Source: three-view drawing plus pictorial views. Frame: mm from the lowest corner of the part. A direction names the side the tool comes from. Give positions to 0.01 mm unless a question says otherwise; leave off trailing zeros. Write each loop counter-clockwise with the first axis right and the second up, starting at its lowest first coordinate (ties: lowest second). Pieces come first, ordered by that corner, then holes. Notation, with made-up numbers: (65.5, 1.25) -> (108.5, 1.25) arc R25 cw to (108.5, 32.25) -> close; hole circle Ø3 at (85.25, 75). An arc over 180 degrees is marked (long way). Write item = value, one per line.
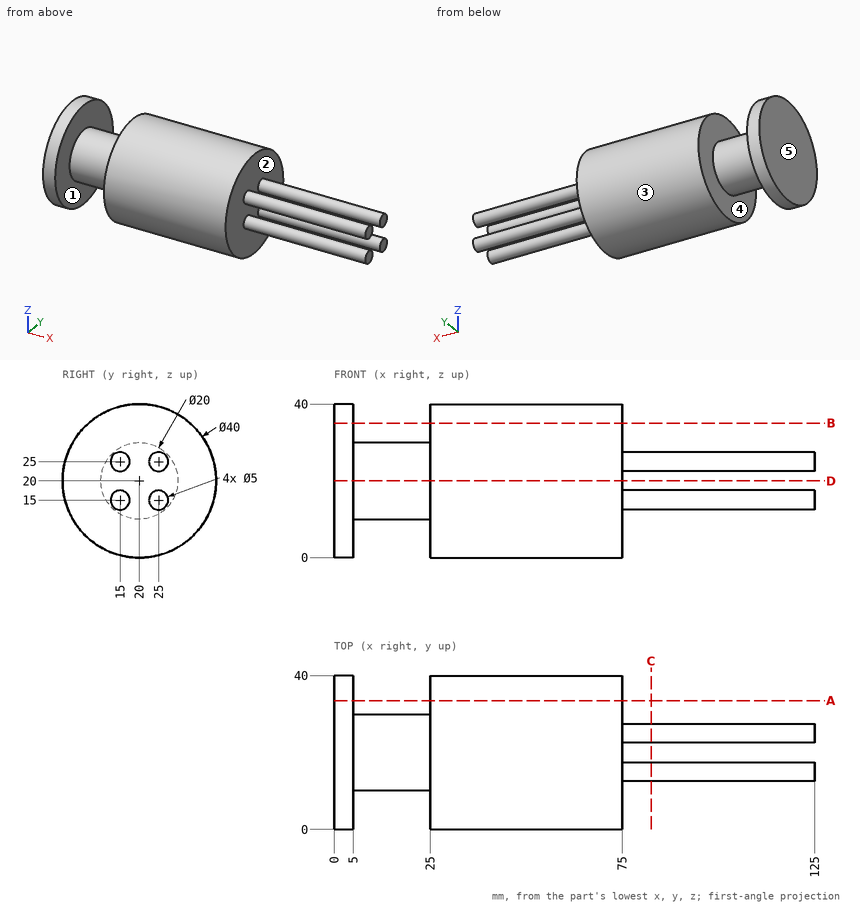
1) Draft query along X for the marked faces 1, 2 and 3. Return one class per face: pulls with the +X half, pulls with the -X half, needs draft (parallel to the pull), parting line crosses it, or undercut.
Computed:
face_1 = undercut
face_2 = pulls with the +X half
face_3 = needs draft
2) Cut plane D-D (z = 20). Return the cut outline in (x, y), then the cut area to 3 significant figures.
Computed:
outline = (0, 0) -> (5, 0) -> (5, 10) -> (25, 10) -> (25, 0) -> (75, 0) -> (75, 40) -> (25, 40) -> (25, 30) -> (5, 30) -> (5, 40) -> (0, 40) -> close
area = 2,600 mm²
3) Cut plane A-A (y = 33.5). Return the cut outline in (x, z), then the cut area to 3 significant figures.
Computed:
outline = (0, 5.24) -> (5, 5.24) -> (5, 34.76) -> (0, 34.76) -> close; (25, 5.24) -> (75, 5.24) -> (75, 34.76) -> (25, 34.76) -> close
area = 1,620 mm²
4) Material intervals for L1, parallel to X at y = 25, z = 9; L2, parallel to Y at x = 31.5, z = 19; L3, parallel to Y at x = 99.5, z = 16, sorted ascending.
Computed:
L1 = 0 to 5, 25 to 75
L2 = 0.03 to 39.97
L3 = 12.71 to 17.29, 22.71 to 27.29
5) Cut plane B-B (z = 35). Return the cut outline in (x, y), then the cut area to 3 significant figures.
Computed:
outline = (0, 6.77) -> (5, 6.77) -> (5, 33.23) -> (0, 33.23) -> close; (25, 6.77) -> (75, 6.77) -> (75, 33.23) -> (25, 33.23) -> close
area = 1,460 mm²
6) Contact query for flat-ended pins moving along their axis: pin 1 (6 mm diameter, centred on x = 64.5, y = 34.5, fed in from -Z); pin 2 (6 mm diameter, centred on y = 12, z = 23, fed in from -X); pin 3 (5 mm diameter, centred on x = 74.5, y = 33, fed in from +Z); pin 4 (1 mm diameter, centred on y = 35, z = 22.5, fed in from +X). Output: stop coordinate, or through.
Computed:
pin_1 = 3.64
pin_2 = 0
pin_3 = 37.02
pin_4 = 75
7) Access query for the marked faces 4 and 5. Directions: +Z, -Z, +X, -X, +Y, -Y. A direction counts if a zero-diameter tool reaches every point of the face in a straight line with its end or side. Return the directions, or none.
Computed:
face_4 = none
face_5 = +Z, -Z, -X, +Y, -Y
8) Cut plane C-C (x = 82.5). Return the cut outline in (y, z), then the cut area to 3 significant figures.
Computed:
outline = circle Ø5 at (15, 15); circle Ø5 at (15, 25); circle Ø5 at (25, 15); circle Ø5 at (25, 25)
area = 78.5 mm²
